```python
from build123d import *


# Read off the part's stored shape, not the designer's step: M14x2.0 Machine Threads Stud1
with BuildPart() as part:
    # Sketch1 → Revolve1 (revolve)
    with BuildSketch(Plane.XY, mode=Mode.PRIVATE) as revolve1_sk:
        Polygon((0, 0), (0, 7.5), (15, 7.5), (15, 3.75), (17, 3.75), (17, 7.5), (47, 7.5), (47, 1.7), (55, 1.7), (55, 0), align=None)
    revolve(revolve1_sk.sketch.rotate(Axis((-20.400760227, 0, 0), (1, 0, 0)), 90), axis=Axis((-20.400760227, 0, 0), (1, 0, 0)))

    # M14x2.0 Machine Threads Stud1 outline → M14x2.0 Machine Threads Stud1 (revolve, cut)
    with BuildSketch(Plane.YX):
        Polygon((7.5, 47), (5.8985, 47), (7, 45.8985), (7, 17), (7.5, 17), align=None)
    revolve(axis=Axis((0, 0, 0), (1, 0, 0)), mode=Mode.SUBTRACT)


solid = part.part
```
Geometry: final body of the model. Coordinates: model frame, mm. A direction names the side the tool comes from. Round coordinates to 2 decimals unless told otherwise and drop trailing zeros. Write each loop counter-clockwise with the first axis right and the second up, starting at its lowest first coordinate (ties: lowest second). Pieces come first, ordered by that corner, then holes.
Item 1: Set-up query: faces 5 (the face through (51.06, 1.66, -0.37)), 6 (the face through (0, 0, 0)), 7 (the face through (15, 3, 3)). Return all of +Z, -Z, +X, -X, +Y, -Y with unobstructed straight access to the full face (end or side cutting, diameter ignored); none if empty.
Item 2: Pin query (flat end, axial travel): P1, Ø8, axis at x = 41.5, z = 0, coming from the +Y side; P2, Ø6, axis at x = 30, y = -1.5, coming from the -Z side; P3, Ø4, axis at x = 44.5, y = 1.5, coming from the +Z side. Return the tip coordinate at first contact, or that it passes through.
Item 3: Material intervals for L1, parallel to X at y = -0.75, z = -4; L2, parallel to Z at x = 29, y = -0.25; L3, parallel to X at y = 3.25, z = -5.5, sorted ascending.
Item 4: Section query A-A (z = 0). Return loops of the section in (x, y).
Item 5: Section query D-D (x = 52). Return loops of the section in (y, z), plus the area to 3 significant figures.
Item 6: Mould query, pull axis X, two halves, no side actions, for faces 1 (the face through (17, 3, -3)), 2 (the face through (16.01, -3.16, 2.02)), 3 (the face through (7.605, -6.324, 4.032)), 4 (the face through (55, 0, 0)). Classes: +X half, -X half, draft (parallel to the pull), parting line (faces both ways), or undercut.
Item 7: Section query C-C (x = 39.5). Return loops of the section in (y, z), plus the area to 3 significant figures.
Completed:
1. face 5: +X
1. face 6: +Z, -Z, -X, +Y, -Y
1. face 7: none
2. P1: stops at y = 7
2. P2: stops at z = -7
2. P3: stops at z = 7
3. L1: x = 0 to 15, 17 to 47
3. L2: z = -7 to 7
3. L3: x = 0 to 15, 17 to 46.51
4. outline: (0, -7.5) - (15, -7.5) - (15, -3.75) - (17, -3.75) - (17, -7) - (45.9, -7) - (47, -5.9) - (47, -1.7) - (55, -1.7) - (55, 1.7) - (47, 1.7) - (47, 5.9) - (45.9, 7) - (17, 7) - (17, 3.75) - (15, 3.75) - (15, 7.5) - (0, 7.5) - close
5. outline: circle Ø3.4 at (0, 0)
5. area: 9.08 mm2
6. face 1: undercut
6. face 2: undercut
6. face 3: draft
6. face 4: +X half
7. outline: circle Ø14 at (0, 0)
7. area: 154 mm2
